Geometry check sheet. Reference: the model listing, model coordinates, mm. A direction names the side the tool comes from. Coordinates: 2 decimals unless noted, no trailing zeros. Write each loop counter-clockwise with the first axis right and the second up, starting at its lowest first coordinate (ties: lowest second). Pieces come first, ordered by that corner, then holes. Notation, with made-up numbers: (44.5, 14) -> (93.5, 14) arc R10 ccw to (93.5, 20) -> close; hole circle Ø8 at (-12, 16). An arc over 180 degrees is marked (long way). One line per question, with ' | ' between items.
```python
from build123d import *

# Parameters (mm, degrees)
SKETCH1_W           = 100
SKETCH1_H           = 70
BOSS_EXTRUDE1_DEPTH = 2.5
SKETCH2_W           = 100
SKETCH2_H           = 5
SKETCH2_H_2         = 3
BOSS_EXTRUDE2_DEPTH = 21
SKETCH3_R           = 7.75
CUT_EXTRUDE1_DEPTH  = 61
BOSS_EXTRUDE3_START = -3
SKETCH4_R           = 7.75
SKETCH4_R_2         = 5
BOSS_EXTRUDE3_DEPTH = 3
SKETCH5_W           = 70
SKETCH5_H           = 2.5
BOSS_EXTRUDE4_DEPTH = 2
SKETCH6_W           = 70
SKETCH6_H           = 2.5
BOSS_EXTRUDE5_DEPTH = 2
CHAMFER1_SIZE       = 5
SKETCH9_W           = 1
SKETCH9_H           = 64
BOSS_EXTRUDE8_DEPTH = 15
CHAMFER3_SIZE       = 2
CHAMFER4_SIZE       = 3
CHAMFER5_SIZE       = 2
SKETCH11_W          = 22
SKETCH11_H          = 31
CUT_EXTRUDE2_DEPTH  = 10
FILLET1_R           = 5


with BuildPart() as part:
    # Sketch1 → Boss-Extrude1 (new body)
    with BuildSketch(Plane(origin=(0, 0, 0), x_dir=(1, 0, 0), z_dir=(0, 1, 0))):
        Rectangle(SKETCH1_W, SKETCH1_H)
    extrude(amount=BOSS_EXTRUDE1_DEPTH)

    # Sketch2 → Boss-Extrude2 (add)
    with BuildSketch(Plane(origin=(0, 2.5, 0), x_dir=(1, 0, 0), z_dir=(0, 1, 0))):
        with Locations((0, 24.5)):
            Rectangle(SKETCH2_W, SKETCH2_H)
        with Locations((0, -24.5)):
            Rectangle(SKETCH2_W, SKETCH2_H_2)
    extrude(amount=BOSS_EXTRUDE2_DEPTH)

    # Sketch3 → Cut-Extrude1 (cut)
    with BuildSketch(Plane(origin=(0, 0, -27), x_dir=(-1, 0, 0), z_dir=(0, 0, -1))):
        with Locations((-33, 13)):
            Circle(SKETCH3_R)
        with Locations((0, 13)):
            Circle(SKETCH3_R)
        with Locations((33, 13)):
            Circle(SKETCH3_R)
    extrude(amount=-CUT_EXTRUDE1_DEPTH, mode=Mode.SUBTRACT)

    # Sketch4 → Boss-Extrude3 (add)
    # profile 1 of 3: a face of its own
    with BuildSketch(Plane.XY.offset(26).offset(BOSS_EXTRUDE3_START)):
        with Locations(Location((-33, 13, 0), (0, 0, 180))):
            Circle(SKETCH4_R)
        with Locations((-33, 13)):
            Circle(SKETCH4_R_2, mode=Mode.SUBTRACT)
    # profile 2 of 3: a face of its own
    with BuildSketch(Plane.XY.offset(26).offset(BOSS_EXTRUDE3_START)):
        with Locations(Location((0, 13, 0), (0, 0, 180))):
            Circle(SKETCH4_R)
        with Locations((0, 13)):
            Circle(SKETCH4_R_2, mode=Mode.SUBTRACT)
    # profile 3 of 3: a face of its own
    with BuildSketch(Plane.XY.offset(26).offset(BOSS_EXTRUDE3_START)):
        with Locations(Location((33, 13, 0), (0, 0, 180))):
            Circle(SKETCH4_R)
        with Locations((33, 13)):
            Circle(SKETCH4_R_2, mode=Mode.SUBTRACT)
    extrude(amount=BOSS_EXTRUDE3_DEPTH)

    # Sketch5 → Boss-Extrude4 (add)
    with BuildSketch(Plane.ZY.offset(50)):
        with Locations((0, 1.25)):
            Rectangle(SKETCH5_W, SKETCH5_H)
    extrude(amount=BOSS_EXTRUDE4_DEPTH)

    # Sketch6 → Boss-Extrude5 (add)
    with BuildSketch(Plane(origin=(50, 0, 0), x_dir=(0, 0, -1), z_dir=(1, 0, 0))):
        with Locations((0, 1.25)):
            Rectangle(SKETCH6_W, SKETCH6_H)
    extrude(amount=BOSS_EXTRUDE5_DEPTH)

    # Chamfer1
    chamfer1_edges = [part.edges().sort_by_distance(p)[0] for p in [
        (52, 1.25, -35),
        (52, 1.25, 35),
        (-50, 23.5, 24.5),
        (50, 23.5, 24.5),
        (-52, 1.25, -35),
        (-52, 1.25, 35),
    ]]
    chamfer(chamfer1_edges, length=CHAMFER1_SIZE)

    # Sketch9 → Boss-Extrude8 (add)
    with BuildSketch(Plane(origin=(0, 2.5, 0), x_dir=(1, 0, 0), z_dir=(0, 1, 0))):
        with Locations((-16.5, 0)):
            Rectangle(SKETCH9_W, SKETCH9_H)
        with Locations((16.5, 0)):
            Rectangle(SKETCH9_W, SKETCH9_H)
    extrude(amount=BOSS_EXTRUDE8_DEPTH)

    # Chamfer3
    chamfer3_edges = [part.edges().sort_by_distance(p)[0] for p in [
        (-16.5, 17.5, -32),
        (-16.5, 17.5, 32),
        (16.5, 17.5, -32),
        (16.5, 17.5, 32),
    ]]
    chamfer(chamfer3_edges, length=CHAMFER3_SIZE)

    # Chamfer4
    chamfer4_edges = [part.edges().sort_by_distance(p)[0] for p in [
        (-50, 23.5, -24.5),
        (50, 23.5, -24.5),
    ]]
    chamfer(chamfer4_edges, length=CHAMFER4_SIZE)

    # Chamfer5
    chamfer5_edges = [part.edges().sort_by_distance(p)[0] for p in [
        (-33.5, 2.5, -22),
        (-33.5, 2.5, 23),
        (0, 2.5, -22),
        (0, 2.5, 23),
        (33.5, 2.5, -22),
        (33.5, 2.5, 23),
    ]]
    chamfer(chamfer5_edges, length=CHAMFER5_SIZE)

    # Sketch11 → Cut-Extrude2 (cut)
    with BuildSketch(Plane(origin=(0, 2.5, 0), x_dir=(1, 0, 0), z_dir=(0, 1, 0))):
        with Locations((0, -0.5)):
            Rectangle(SKETCH11_W, SKETCH11_H)
        with Locations((-33, -0.5)):
            Rectangle(SKETCH11_W, SKETCH11_H)
        with Locations((33, -0.5)):
            Rectangle(SKETCH11_W, SKETCH11_H)
    extrude(amount=-CUT_EXTRUDE2_DEPTH, mode=Mode.SUBTRACT)

    # Fillet1
    fillet1_edges = [part.edges().sort_by_distance(p)[0] for p in [
        (-11, 1.25, 16),
        (-11, 1.25, -15),
        (11, 1.25, -15),
        (11, 1.25, 16),
        (-22, 1.25, -15),
        (-22, 1.25, 16),
        (-44, 1.25, 16),
        (-44, 1.25, -15),
        (22, 1.25, 16),
        (22, 1.25, -15),
        (44, 1.25, -15),
        (44, 1.25, 16),
    ]]
    fillet(fillet1_edges, radius=FILLET1_R)


solid = part.part
```
(1) Cross-section at A-A (z = -1). Record the cut outline in (x, y).
Answers below:
outline: (-52, 0) -> (-44, 0) -> (-44, 2.5) -> (-52, 2.5) -> close; (-22, 0) -> (-11, 0) -> (-11, 2.5) -> (-16, 2.5) -> (-16, 17.5) -> (-17, 17.5) -> (-17, 2.5) -> (-22, 2.5) -> close; (11, 0) -> (22, 0) -> (22, 2.5) -> (17, 2.5) -> (17, 17.5) -> (16, 17.5) -> (16, 2.5) -> (11, 2.5) -> close; (44, 0) -> (52, 0) -> (52, 2.5) -> (44, 2.5) -> close
(2) Depth check by flat-ended pin: P1, Ø13, axis at x = -33, y = 13, coming from the -Z side; P2, Ø5, axis at y = 9.5, z = 30.5, coming from the -X side; P3, Ø0.5, axis at x = 16.5, y = 12, coming from the +Z side; P4, Ø1, axis at x = 31.5, y = 9.5, coming from the -Z side. Enter the tip coordinate at first touch or a pass-through.
Answers below:
P1: stops at z = 23 | P2: stops at x = -17 | P3: stops at z = 32 | P4: passes through
(3) Cross-section at C-C (y = 13). Count the separate pieces of the cut face and the enclosed holes in it, plus the area to 4 significant figures.
Answers below:
separate pieces: 6 | enclosed holes: 0 | area: 589.5 mm²
(4) Cross-section at D-D (z = 14). Record the cut outline in (x, y), plus the area to 3 significant figures.
Answers below:
outline: (-52, 0) -> (-43, 0) -> (-43, 2.5) -> (-52, 2.5) -> close; (-23, 0) -> (-10, 0) -> (-10, 2.5) -> (-16, 2.5) -> (-16, 17.5) -> (-17, 17.5) -> (-17, 2.5) -> (-23, 2.5) -> close; (10, 0) -> (23, 0) -> (23, 2.5) -> (17, 2.5) -> (17, 17.5) -> (16, 17.5) -> (16, 2.5) -> (10, 2.5) -> close; (43, 0) -> (52, 0) -> (52, 2.5) -> (43, 2.5) -> close | area: 140 mm²
(5) Tool access check on faces 4 (the face through (33, 1, -15)), 5 (the face through (-17, 10, 29)), 6 (the face through (1, 20, 23)). Record the directions out of +Z, -Z, +X, -X, +Y, -Y that give a thin tool (end or side, any length) a straight path to the whole face; none if there is none.
Answers below:
face 4: +Y, -Y | face 5: +Z, -X, +Y | face 6: +Y
(6) Cross-section at B-B (x = 0). Record the cut outline in (y, z), plus the area to 3 significant figures.
Answers below:
outline: (0, -35) -> (2.5, -35) -> (2.5, -27) -> (5.25, -27) -> (5.25, -22) -> (4.5, -22) -> (2.5, -20) -> (2.5, -15) -> (0, -15) -> close; (0, 16) -> (2.5, 16) -> (2.5, 21) -> (4.5, 23) -> (8, 23) -> (8, 26) -> (2.5, 26) -> (2.5, 35) -> (0, 35) -> close; (18, 23) -> (23.5, 23) -> (23.5, 26) -> (18, 26) -> close; (20.75, -27) -> (23.5, -27) -> (23.5, -22) -> (20.75, -22) -> close | area: 162 mm²
(7) Material ranges on line 1 (Z direction, x = -20, y = 20.25); line 2 (X direction, y = 12.75, z = 12); line 3 (Y direction, x = 0, z = -24.2), recorded low to high.
Answers below:
line 1: z = -27 to -22, 23 to 26 | line 2: x = -17 to -16, 16 to 17 | line 3: y = 0 to 5.25, 20.75 to 23.5
(8) Draft check along Z on faces 1 (the face through (44, 1, 1)), 2 (the face through (-50, 11, -24)), 3 (the face through (-1, 1, 35)). Enter one of: pulls with the +Z half, pulls with the -Z half, needs draft (parallel to the pull), parting line crosses it, or undercut.
Answers below:
face 1: undercut | face 2: needs draft | face 3: pulls with the +Z half
